from build123d import *

# Parameters (mm, degrees)
SKETCH_1_W      = 7
SKETCH_1_H      = 230
SKETCH_1_R      = 1.25
EXTRUDE_1_DEPTH = 4.8


with BuildPart() as part:
    # 草图1 → 凸台-拉伸1 (new body)
    with BuildSketch(Plane(origin=(0, 0, 0), x_dir=(1, 0, 0), z_dir=(0, 1, 0))):
        Rectangle(SKETCH_1_W, SKETCH_1_H)
        with Locations(Location((0, 107.5, 0), (0, 0, 270))):
            Circle(SKETCH_1_R, mode=Mode.SUBTRACT)
        with Locations(Location((0, 92.5, 0), (0, 0, 270))):
            Circle(SKETCH_1_R, mode=Mode.SUBTRACT)
        with Locations(Location((0, 77.5, 0), (0, 0, 270))):
            Circle(SKETCH_1_R, mode=Mode.SUBTRACT)
        with Locations(Location((0, 62.5, 0), (0, 0, 270))):
            Circle(SKETCH_1_R, mode=Mode.SUBTRACT)
        with Locations(Location((0, 47.5, 0), (0, 0, 270))):
            Circle(SKETCH_1_R, mode=Mode.SUBTRACT)
        with Locations(Location((0, 32.5, 0), (0, 0, 270))):
            Circle(SKETCH_1_R, mode=Mode.SUBTRACT)
        with Locations(Location((0, 17.5, 0), (0, 0, 270))):
            Circle(SKETCH_1_R, mode=Mode.SUBTRACT)
        with Locations(Location((0, 2.5, 0), (0, 0, 270))):
            Circle(SKETCH_1_R, mode=Mode.SUBTRACT)
        with Locations(Location((0, -12.5, 0), (0, 0, 270))):
            Circle(SKETCH_1_R, mode=Mode.SUBTRACT)
        with Locations(Location((0, -27.5, 0), (0, 0, 270))):
            Circle(SKETCH_1_R, mode=Mode.SUBTRACT)
        with Locations(Location((0, -42.5, 0), (0, 0, 270))):
            Circle(SKETCH_1_R, mode=Mode.SUBTRACT)
        with Locations(Location((0, -57.5, 0), (0, 0, 270))):
            Circle(SKETCH_1_R, mode=Mode.SUBTRACT)
        with Locations(Location((0, -72.5, 0), (0, 0, 270))):
            Circle(SKETCH_1_R, mode=Mode.SUBTRACT)
        with Locations(Location((0, -87.5, 0), (0, 0, 270))):
            Circle(SKETCH_1_R, mode=Mode.SUBTRACT)
        with Locations(Location((0, -102.5, 0), (0, 0, 270))):
            Circle(SKETCH_1_R, mode=Mode.SUBTRACT)
    extrude(amount=EXTRUDE_1_DEPTH)


solid = part.part
Can you work these out from the model? Positions are in its coordinate system, mm. Give positions to 0.01 mm unless a question says otherwise; leave off trailing zeros. Use one line per item in the form item = value. Start each with the question number.
Item 1: If I drill on line 1 along X through (y, z) = (1.35, -107.5); line 2 along X through (y, z) = (2.95, -31.5), over which ranges is the centre line in solid material (lowest first)?
Item 2: If we section it at A-A (y = 3.5): State how many separate pieces and enclosed holes the cut face has, then the cut area to 3 significant figures.
Item 3: Will this pin go through, and if not, where does the flat tip stop? pin 1 Ø2 at (x, z) = (0, -47.5) entering from -Y.
Outcome:
q1.line_1 = -3.5 to -1.25, 1.25 to 3.5
q1.line_2 = -3.5 to -0.75, 0.75 to 3.5
q2.separate_pieces = 1
q2.enclosed_holes = 15
q2.area = 1,540 mm2
q3.pin_1 = through
